Could you check a few things on this drawing? It's one solid part, dimensions in mm from its lowest x, y, z. A direction names the side the tool comes from. Round coordinates to 2 decimals unless told otherwise and drop trailing zeros. Order: outer loops, then holes, each group sorted by start corner. A loop starts at its lowest first (then second) coordinate and runs counter-clockwise, first axis right, second up. Notation, with made-up numbers: M 65,-20.5 L 108,-20.5 A11 ccw 108,-9.5 Z; hole C -13,76 d10. An arc over 180 degrees is marked long. Answer as CSV lines item,"result". Start each with the question number.
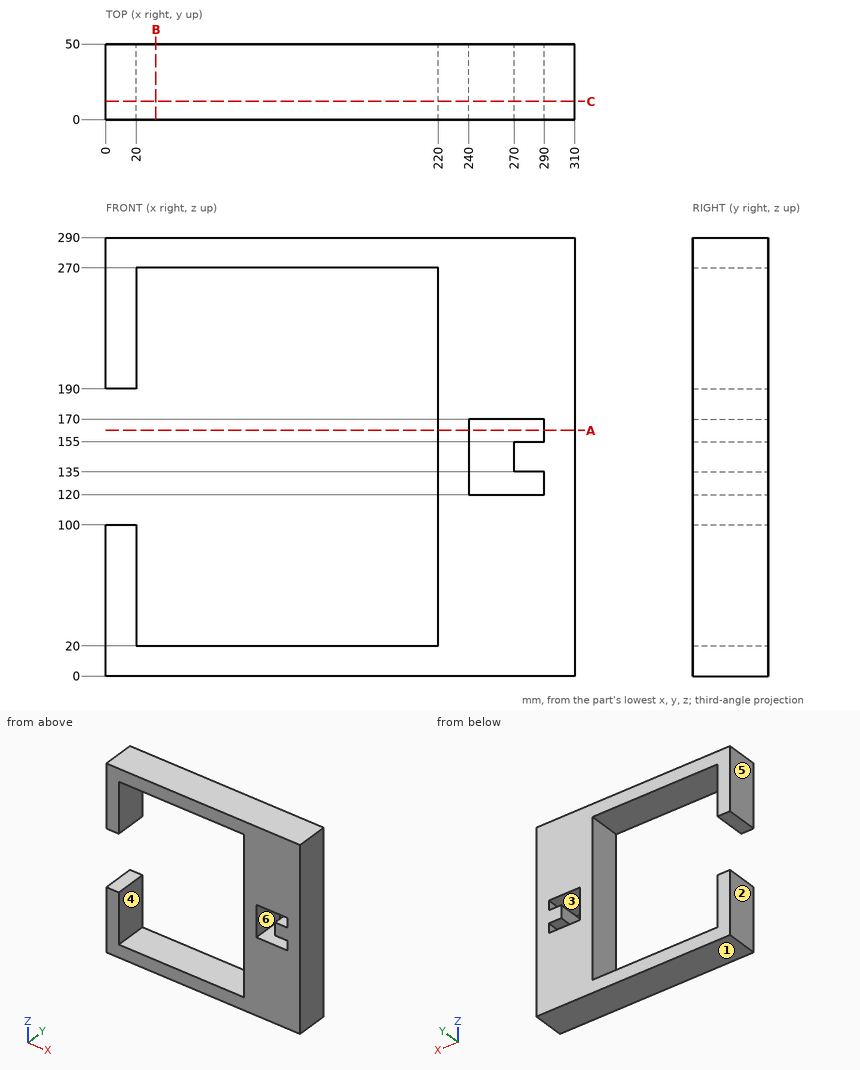
Item 1: If I drill on line 1 along Z through (x, y) = (276, 27); line 2 along Z through (x, y) = (124, 39); line 3 along X through (y, z) = (21.5, 74), over which ranges is the centre line in solid material (lowest first)?
Item 2: If we section it at A-A on z = 162.5: Please give me the cut outline in (x, y), and give its area (3 significant figures).
Item 3: For P1, Ø12, axis at y = 16.5, z = 160.5, coming from the -X side, with a flat end and sliding along its axis, tell me the tip position at first contact or that it passes through.
Item 4: If we section it at B-B on x = 33: Please give me the cut outline in (y, z).
Item 5: We'd pull the mould along X, two halves only. Please class the marked faces 1, 2, 3 and 4: pulls with the +X half, pulls with the -X half, needs draft (parallel to the pull), parting line crosses it, or undercut.
Item 6: Which directions (+Z, -Z, +X, -X, +Y, -Y) give clear straight access to the entire face, cutting with the end or side of a thin tool? Please do the marked faces 5 and 6.
Item 7: If we section it at C-C on y = 12: Please give me the cut outline in (x, z), and give its area (3 significant figures).
Geometry says:
1,line 1,"0 to 120, 135 to 155, 170 to 290"
1,line 2,"0 to 20, 270 to 290"
1,line 3,"0 to 20, 220 to 310"
2,outline,"M 220,0 L 240,0 L 240,50 L 220,50 Z; M 290,0 L 310,0 L 310,50 L 290,50 Z"
2,area,"2,000 mm²"
3,P1,"x = 220"
4,outline,"M 0,0 L 50,0 L 50,20 L 0,20 Z; M 0,270 L 50,270 L 50,290 L 0,290 Z"
5,face 1,"needs draft"
5,face 2,"pulls with the -X half"
5,face 3,"undercut"
5,face 4,"undercut"
6,face 5,"+Z, -Z, -X, +Y, -Y"
6,face 6,"+Y, -Y"
7,outline,"M 0,0 L 310,0 L 310,290 L 0,290 L 0,190 L 20,190 L 20,270 L 220,270 L 220,20 L 20,20 L 20,100 L 0,100 Z; hole M 240,120 L 290,120 L 290,135 L 270,135 L 270,155 L 290,155 L 290,170 L 240,170 Z"
7,area,"36,000 mm²"
